Build history of the part. All positions in model axes, mm. A direction names the side the tool comes from. Round coordinates to 2 decimals unless told otherwise and drop trailing zeros. Write each loop counter-clockwise with the first axis right and the second up, starting at its lowest first coordinate (ties: lowest second). Pieces come first, ordered by that corner, then holes. Notation, with made-up numbers: (60.25, 65) -> (93.25, 65) arc R17 cw to (93.25, 81) -> close; hole circle Ø8 at (-2, -31). An arc over 180 degrees is marked (long way). Return JSON: item names as keys, results as strings.
Autodesk Inventor part; units mm, degrees
ref_plane "YZ Plane" through (0, 0, 0) normal (1, 0, 0) x (0, 1, 0)
ref_plane "XZ Plane" through (0, 0, 0) normal (0, 1, 0) x (-1, 0, 0)
ref_plane "XY Plane" through (0, 0, 0) normal (0, 0, 1) x (1, 0, 0)
sketch "Sketch1" plane through (0, 0, 0) normal (0, 0, 1) x (1, 0, 0)
  arc A0 (-3.175, 12.7) -> (3.175, 12.7) centre (0, 12.7) ccw
  line L0 (0, -1.6305) -> (0, 0) construction
  line L1 (0, -1.6305) -> (0, 9.525) construction
  line L2 (3.175, 12.7) -> (3.175, 14.2875)
  line L3 (3.175, 14.2875) -> (4.7625, 14.2875)
  line L4 (4.7625, 14.2875) -> (4.7625, 9.525)
  line L5 (-3.175, 12.7) -> (-3.175, 14.2875)
  line L6 (-3.175, 14.2875) -> (-4.7625, 14.2875)
  line L7 (-4.7625, 14.2875) -> (-4.7625, 9.525)
  line L8 (9.525, 3.175) -> (-9.525, 3.175)
  line L9 (3.175, 12.7) -> (-3.175, 12.7) construction
  line L10 (9.525, 6.35) -> (9.525, 3.175)
  line L11 (-9.525, 6.35) -> (-9.525, 3.175)
  line L12 (9.525, 6.35) -> (4.7625, 9.525)
  line L13 (-4.7625, 9.525) -> (-9.525, 6.35)
  line L14 (21.4144, 0) -> (-14.6121, 0) construction
  point P0 (0, 3.175)
  dimension "d1" = 1.5875
  dimension "d2" = 1.5875
  dimension "d7" = 9.525
  dimension "d8" = 3.175
  dimension "d10" = 3.175
  dimension "d11" = 9.525
  dimension "d12" = 19.05
  dimension "d13" = 3.175
  dimension "d14" = 3.175
revolve "Revolution1" add sketch "Sketch1" angle 360 about axis through (21.4144, 0, 0) along (-1, 0, 0)
sketch "Sketch2" plane through (0, 0, 0) normal (1, 0, 0) x (0, 1, 0)
  circle A0 centre (0, 0) radius 3.175
  circle A1 centre (0, 0) radius 7.9375
  point P0 (0, 0)
  dimension "d16" = 15.875
extrude "Extrusion1" cut sketch "Sketch2" along normal mid plane 6.35
properties part number "line pulley" material "ABS Plastic"
Q1. Two-plate mould, pull along X, no slides. Class faces 1 (the flat face through (-4.762, 3, 9.3)), 2 (the flat face through (3.175, -13, 1)), 3 (the cylindrical face through (3.98, -14.274, 0.628)): +X half, -X half, draft (parallel to the pull), parting line (faces both ways), or undercut.
Verdict:
{"face 1": "-X half", "face 2": "undercut", "face 3": "draft"}
Q2. Wall check: L1, parallel to X at y = 4, z = 0.25 (3 decimals); L2, parallel to Z at x = -7, y = 0 (3 decimals); L3, parallel to X at y = -7.25, z = 0.75 (3 decimals). Give the ranges that are in metal, low to high.
Verdict:
{"L1": "x = -9.525 to -3.175, 3.175 to 9.525", "L2": "z = -8.033 to -3.175, 3.175 to 8.033", "L3": "x = -8.117 to -3.175, 3.175 to 8.117"}
Q3. Saw through at C-C on x = -6.25. List the corners of the cut face in (y, z) (3 decimals), then the cut area to 3 significant figures.
Verdict:
{"outline": "circle Ø17.067 at (0, 0); hole circle Ø6.35 at (0, 0)", "area": "197 mm²"}
Q4. 3-axis set-ups, long thin cutter, end or side, ignore diameter. For faces 4 (the flat face through (3.175, 3.4, 0.1)), 5 (the flat face through (4.762, 3, 9.3)), 6 (the cylindrical face through (-3.98, -14.274, -0.628)): which of +Z, -Z, +X, -X, +Y, -Y reach the whole face in a straight line?
Verdict:
{"face 4": "none", "face 5": "+X", "face 6": "+X, -X"}
Q5. Pin check, flat tips, straight feed: pin 1 Ø10 at (x, y) = (-3.5, 8.5) entering from -Z; pin 2 Ø5 at (x, y) = (-3.5, 4) entering from -Z; pin 3 Ø1 at (y, z) = (-8.5, -4) entering from +X; pin 4 Ø9.5 at (y, z) = (0, 0) entering from -X (3 decimals). Stop position of each tip, or through.
Verdict:
{"pin 1": "stops at z = -13.85", "pin 2": "stops at z = -14.21", "pin 3": "stops at x = 5.71", "pin 4": "stops at x = -9.525"}
